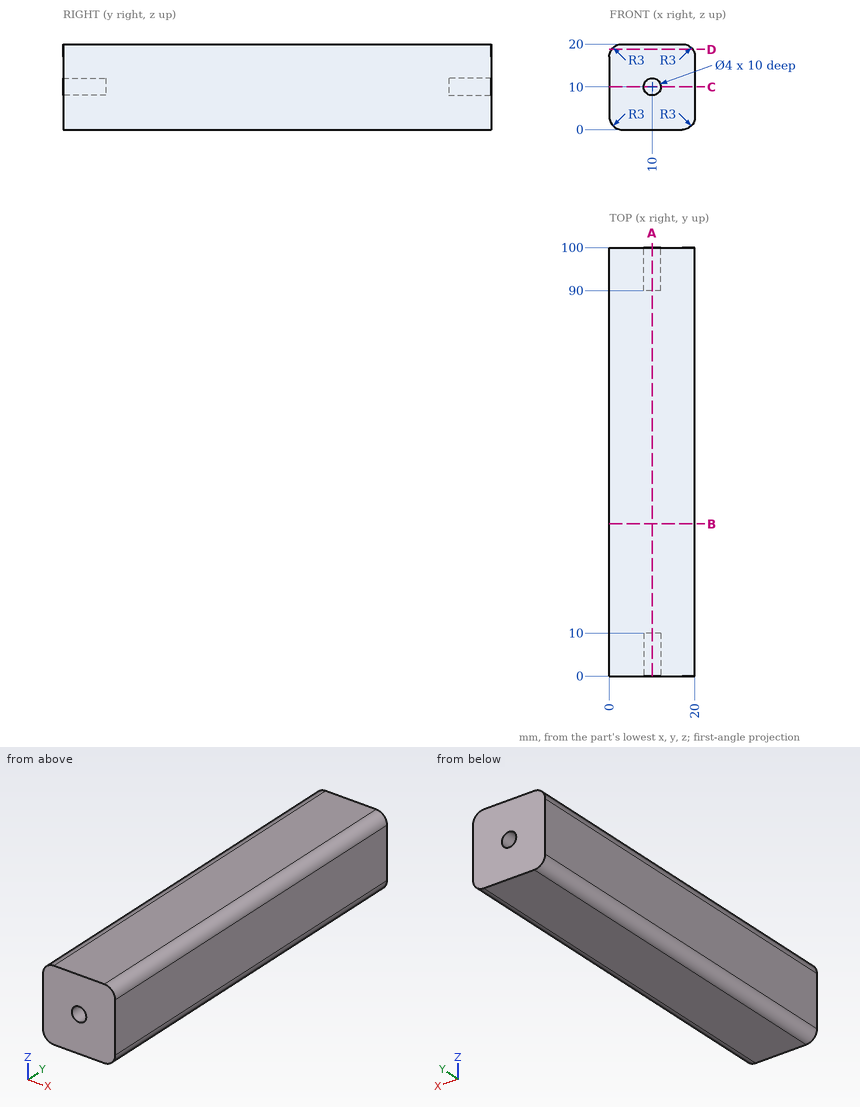
Input: dimensioned drawing with shaded views. Units: mm. Origin: part minimum x, y, z. Round coordinates to 2 decimals unless told otherwise and drop trailing zeros. Order: outer loops, then holes, each group sorted by start corner. A loop starts at its lowest first (then second) coordinate and runs counter-clockwise, first axis right, second up.
1. Material intervals for line 1 (X direction, y = 96.5, z = 10); line 2 (X direction, y = 14, z = 2); line 3 (Z direction, x = 18.5, y = 11), sorted ascending.
The answers:
line 1: x = 0 to 8, 12 to 20
line 2: x = 0.17 to 19.83
line 3: z = 0.4 to 19.6
2. Pin query (flat end, axial travel): P1, Ø8, axis at x = 11, z = 2, coming from the -Y side; P2, Ø3, axis at x = 10, z = 10, coming from the -Y side. Return the tip coordinate at first contact, or that it passes through.
The answers:
P1: stops at y = 0
P2: stops at y = 10
3. Cut plane C-C, the plane z = 10. Output: boundary loops of the cut face in (x, y).
The answers:
outline: (0, 0) - (8, 0) - (8, 10) - (12, 10) - (12, 0) - (20, 0) - (20, 100) - (12, 100) - (12, 90) - (8, 90) - (8, 100) - (0, 100) - close
4. Cut plane D-D, the plane z = 18.75. Output: boundary loops of the cut face in (x, y).
The answers:
outline: (0.56, 0) - (19.44, 0) - (19.44, 100) - (0.56, 100) - close
5. Cut plane B-B, the plane y = 35.5. Output: boundary loops of the cut face in (x, z), then the cut area to 3 significant figures.
The answers:
outline: (0, 3) arc R3 ccw to (3, 0) - (17, 0) arc R3 ccw to (20, 3) - (20, 17) arc R3 ccw to (17, 20) - (3, 20) arc R3 ccw to (0, 17) - close
area: 392 mm2
6. Cut plane A-A, the plane x = 10. Output: boundary loops of the cut face in (y, z), then the cut area to 3 significant figures.
The answers:
outline: (0, 0) - (100, 0) - (100, 8) - (90, 8) - (90, 12) - (100, 12) - (100, 20) - (0, 20) - (0, 12) - (10, 12) - (10, 8) - (0, 8) - close
area: 1,920 mm2
